Geometry: see drawing. Coordinates: mm, zero at the bounding-box minimum. A direction names the side the tool comes from. Give positions to 0.01 mm unless a question says otherwise; leave off trailing zeros. Write each loop counter-clockwise with the first axis right and the second up, starting at its lowest first coordinate (ties: lowest second). Pieces come first, ordered by that corner, then holes.
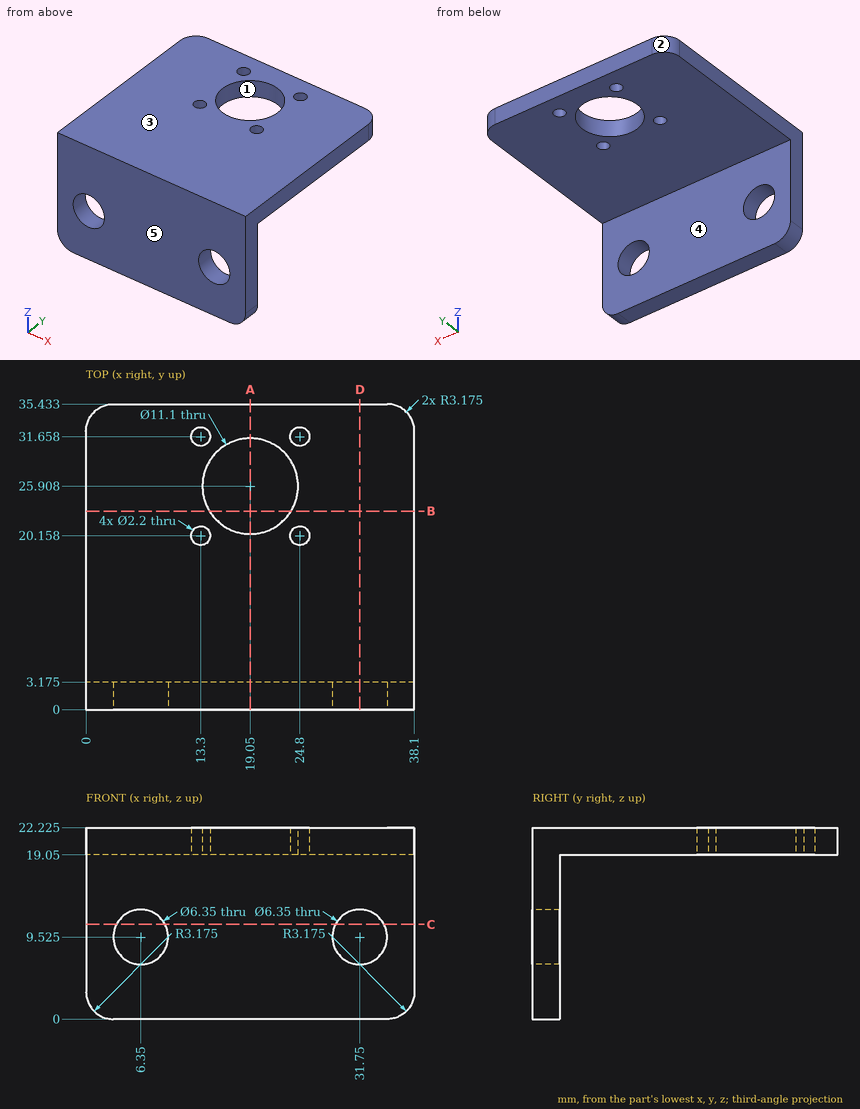
Q1. Section C-C, the plane z = 11. Return the cut outline in (x, y) (3 decimals), then the cut area to 3 significant figures.
Q2. Pin query (flat end, axial travel): pin 1 (7.5 mm diameter, centred on x = 31.75, z = 9.525, fed in from +Y) (3 decimals); pin 2 (3 mm diameter, centred on x = 13.3, y = 31.658, fed in from -Z). Return the tip coordinate at first contact, or that it passes through.
Q3. Material intervals for line 1 along Y through (x, z) = (24.8, 21.35); line 2 along Y through (x, z) = (19.05, 21.2); line 3 along X through (y, z) = (2, 10.5), sorted ascending.
Q4. Mould query, pull axis Y, two halves, no side actions, for the marked faces 1, 2 and 3. Classes: +Y half, -Y half, draft (parallel to the pull), parting line (faces both ways), or undercut.
Q5. Access query for the marked faces 4 and 5. Directions: +Z, -Z, +X, -X, +Y, -Y. A direction counts if a zero-diameter tool reaches every point of the face in a straight line with its end or side. Return the directions, or none.
Q6. Section B-B, the plane y = 23. Return the cut outline in (x, z) (3 decimals), then the cut area to 4 significant figures.
Q7. Section D-D, the plane x = 31.75. Return the cut outline in (y, z) (3 decimals).
Q8. Section A-A, the plane x = 19.05. Return the cut outline in (y, z) (3 decimals), then the cut area to 3 significant figures.
Solutions:
1. outline: (0, 0) - (3.538, 0) - (3.538, 3.175) - (0, 3.175) - close; (9.162, 0) - (28.938, 0) - (28.938, 3.175) - (9.162, 3.175) - close; (34.562, 0) - (38.1, 0) - (38.1, 3.175) - (34.562, 3.175) - close
1. area: 85.3 mm2
2. pin 1: stops at y = 3.175
2. pin 2: stops at z = 19.05
3. line 1: y = 0 to 19.06, 21.26 to 30.56, 32.76 to 35.43
3. line 2: y = 0 to 20.36, 31.46 to 35.43
3. line 3: x = 0 to 3.33, 9.37 to 28.73, 34.77 to 38.1
4. face 1: undercut
4. face 2: +Y half
4. face 3: draft
5. face 4: -Z, +X, -X, +Y
5. face 5: +Z, -Z, +X, -X, -Y
6. outline: (0, 19.05) - (14.323, 19.05) - (14.323, 22.225) - (0, 22.225) - close; (23.777, 19.05) - (38.1, 19.05) - (38.1, 22.225) - (23.777, 22.225) - close
6. area: 90.95 mm2
7. outline: (0, 0) - (3.175, 0) - (3.175, 6.35) - (0, 6.35) - close; (0, 12.7) - (3.175, 12.7) - (3.175, 19.05) - (35.433, 19.05) - (35.433, 22.225) - (0, 22.225) - close
8. outline: (0, 0) - (3.175, 0) - (3.175, 19.05) - (20.358, 19.05) - (20.358, 22.225) - (0, 22.225) - close; (31.458, 19.05) - (35.433, 19.05) - (35.433, 22.225) - (31.458, 22.225) - close
8. area: 138 mm2
